```python
from build123d import *

# Parameters (mm, degrees)
SKETCH1_R           = 16
SKETCH1_R_2         = 13
SKETCH1_R_3         = 2.75
BOSS_EXTRUDE1_DEPTH = 3.5
FILLET2_R           = 2
FILLET3_R           = 2
SKETCH4_R           = 14
CUT_EXTRUDE2_DEPTH  = 0.1


with BuildPart() as part:
    # Sketch1 → Boss-Extrude1 (new body, symmetric)
    with BuildSketch(Plane(origin=(0, 0, 0), x_dir=(1, 0, 0), z_dir=(0, 1, 0))):
        Circle(SKETCH1_R)
        Circle(SKETCH1_R_2, mode=Mode.SUBTRACT)
        with BuildLine():
            ThreePointArc((-2.106622219, -1.767665927), (-2.38156986, -1.375), (-2.584154707, -0.940555394))
            Line((-2.584154707, -0.940555394), (-12.21600407, -4.446261863))
            ThreePointArc((-12.21600407, -4.446261863), (-11.258330249, -6.5), (-9.958577761, -8.356238926))
            Line((-9.958577761, -8.356238926), (-2.106622219, -1.767665927))
        make_face()
        Circle(SKETCH1_R_3)
        with BuildLine():
            ThreePointArc((-1.227230113, 0.8625), (0, -1.5), (1.227230113, 0.8625))
            Line((1.227230113, 0.8625), (-1.227230113, 0.8625))
        make_face(mode=Mode.SUBTRACT)
        with BuildLine():
            Line((-2.25742631, 12.802500789), (-0.477532489, 2.708221321))
            ThreePointArc((-0.477532489, 2.708221321), (0, 2.75), (0.477532489, 2.708221321))
            Line((0.477532489, 2.708221321), (2.25742631, 12.802500789))
            ThreePointArc((2.25742631, 12.802500789), (0, 13), (-2.25742631, 12.802500789))
        make_face()
        with BuildLine():
            Line((12.21600407, -4.446261863), (2.584154707, -0.940555394))
            ThreePointArc((2.584154707, -0.940555394), (2.38156986, -1.375), (2.106622219, -1.767665927))
            Line((2.106622219, -1.767665927), (9.958577761, -8.356238926))
            ThreePointArc((9.958577761, -8.356238926), (11.258330249, -6.5), (12.21600407, -4.446261863))
        make_face()
    extrude(amount=BOSS_EXTRUDE1_DEPTH, both=True)

    # Fillet2
    fillet2_edges = [part.edges().sort_by_distance(p)[0] for p in [
        (-16, -3.5, 0),
        (-16, 3.5, 0),
    ]]
    fillet(fillet2_edges, radius=FILLET2_R)

    # Fillet3
    fillet3_edges = [part.edges().sort_by_distance(p)[0] for p in [
        (2.584154707, 0, 0.940555394),
        (12.21600407, 0, 4.446261863),
        (2.25742631, 0, -12.802500789),
        (0.477532489, 0, -2.708221321),
        (-2.25742631, 0, -12.802500789),
        (-12.21600407, 0, 4.446261863),
        (-2.584154707, 0, 0.940555394),
        (-0.477532489, 0, -2.708221321),
        (-9.958577761, 0, 8.356238926),
        (9.958577761, 0, 8.356238926),
        (2.106622219, 0, 1.767665927),
        (-2.106622219, 0, 1.767665927),
    ]]
    fillet(fillet3_edges, radius=FILLET3_R)

    # Sketch4 → Cut-Extrude2 (cut)
    with BuildSketch(Plane(origin=(0, 3.5, 0), x_dir=(1, 0, 0), z_dir=(0, 1, 0))):
        Circle(SKETCH4_R)
    cut_extrude2 = extrude(amount=-CUT_EXTRUDE2_DEPTH, mode=Mode.SUBTRACT)

    # Mirror1: Cut-Extrude2 across plane
    add(cut_extrude2.mirror(Plane.ZX), mode=Mode.SUBTRACT)


solid = part.part
```
CAD build for the part. Positions are in the model's coordinates, mm. A direction names the side the tool comes from. Round coordinates to 2 decimals unless told otherwise and drop trailing zeros. Loops run counter-clockwise (first coordinate to the right, second up) from the corner with the lowest first, then second, coordinate; pieces in that order, holes last. Notation, with made-up numbers: M 63.25,88 L 83.25,88 A11 cw 83.25,93 Z; hole C 0.25,-3.5 d5. An arc over 180 degrees is marked long. Use a Markdown table: item, result. Add a question column.
(1) Cut at A-A (x = 0). Give the cut face in (y, z).
(2) Cut at C-C (y = 2.75). Give the cut face in (x, z), and give its area (3 significant figures).
(3) Cut at D-D (x = -6). State how many separate pieces and enclosed holes the cut face has, and give its area (3 significant figures).
(4) Flat gauge pins, fed straight in: pin 1 (1.5 mm diameter, centred on y = 1.5, z = 10, fed in from +X); pin 2 (8.5 mm diameter, centred on x = 2, z = 1, fed in from +Y); pin 3 (4 mm diameter, centred on x = 0, z = 0, fed in from -Y). Where does each tip first touch, or does it go through?
(5) Drill centre lines: line 1 (X direction, y = 2.5, z = 1); line 2 (X direction, y = -2, z = -3); line 3 (X direction, y = -3, z = -1.5). Where is each one in solid material? Low to high.
(6) Cut at B-B (y = -2). Give the cut face in (x, z).
(7) Pull direction Z, two halves, no side cores. Call faces 1 (the face through (0, 0, -0.862)), 2 (the face through (-3.47, 0.02, 15.62)), 3 (the face through (2.876, -0.048, -12.053)): +Z half, -Z half, draft (parallel to the pull), parting line (faces both ways), or undercut.
(8) Which spindle directions (+Z, -Z, +X, -X, +Y, -Y) get a long thin tool onto all of the face, cutting with end or side? Do faces 4 (the face through (-0.1, -3.4, -1.1)), 5 (the face through (-2.876, 0.048, -12.053)), 6 (the face through (-0.1, 3.4, -1.1)). Say none if no direction does.
Geometry says:
| question | item | result |
|---|---|---|
| 1 | outline | M -3.5,-14 A2 ccw -1.5,-16 L 1.5,-16 A2 ccw 3.5,-14 L 3.4,-14 L 3.4,-0.86 L -3.4,-0.86 L -3.4,-14 Z; M -3.5,14 L -3.4,14 L -3.4,13 L 3.4,13 L 3.4,14 L 3.5,14 A2 ccw 1.5,16 L -1.5,16 A2 ccw Z; M -3.4,1.5 L 3.4,1.5 L 3.4,2.75 L -3.4,2.75 Z |
| 2 | outline | C 0,0 d31.12; hole M -12.82,2.15 A13 ccw -4.55,-12.18 A2 ccw -1.88,-10.65 L -0.75,-4.24 A2 ccw -1.57,-2.26 A2.75 cw -2.74,-0.23 A2 ccw -4.05,1.47 L -10.16,3.7 A2 ccw Z; hole M -8.29,6.95 L -3.3,2.77 A2 ccw -1.17,2.49 A2.75 cw 1.17,2.49 A2 ccw 3.3,2.77 L 8.29,6.95 A2 ccw 8.27,10.03 A13 ccw -8.27,10.03 A2 ccw Z; hole M -1.23,-0.86 L 1.23,-0.86 A1.5 ccw long Z; hole M 0.75,-4.24 L 1.88,-10.65 A2 ccw 4.55,-12.18 A13 ccw 12.82,2.15 A2 ccw 10.16,3.7 L 4.05,1.47 A2 ccw 2.74,-0.23 A2.75 cw 1.57,-2.26 A2 ccw Z |
| 2 | area | 341 mm² |
| 3 | separate pieces | 3 |
| 3 | enclosed holes | 0 |
| 3 | area | 61.4 mm² |
| 4 | pin 1 | stops at x = 13.06 |
| 4 | pin 2 | stops at y = 3.4 |
| 4 | pin 3 | stops at y = -3.4 |
| 5 | line 1 | x = -15.7 to -12.96, -3.31 to -1.12, 1.12 to 3.31, 12.96 to 15.7 |
| 5 | line 2 | x = -15.65 to -12.65, -0.93 to 0.93, 12.65 to 15.65 |
| 5 | line 3 | x = -15.25 to -12.91, -2.3 to 2.3, 12.91 to 15.25 |
| 6 | outline | C 0,0 d31.87; hole M -12.82,2.15 A13 ccw -4.55,-12.18 A2 ccw -1.88,-10.65 L -0.75,-4.24 A2 ccw -1.57,-2.26 A2.75 cw -2.74,-0.23 A2 ccw -4.05,1.47 L -10.16,3.7 A2 ccw Z; hole M -8.29,6.95 L -3.3,2.77 A2 ccw -1.17,2.49 A2.75 cw 1.17,2.49 A2 ccw 3.3,2.77 L 8.29,6.95 A2 ccw 8.27,10.03 A13 ccw -8.27,10.03 A2 ccw Z; hole M -1.23,-0.86 L 1.23,-0.86 A1.5 ccw long Z; hole M 0.75,-4.24 L 1.88,-10.65 A2 ccw 4.55,-12.18 A13 ccw 12.82,2.15 A2 ccw 10.16,3.7 L 4.05,1.47 A2 ccw 2.74,-0.23 A2.75 cw 1.57,-2.26 A2 ccw Z |
| 7 | face 1 | undercut |
| 7 | face 2 | parting line |
| 7 | face 3 | undercut |
| 8 | face 4 | -Y |
| 8 | face 5 | +Y, -Y |
| 8 | face 6 | +Y |
